from build123d import *

# Parameters (mm, degrees)
F0_W        = 2
F0_H        = 7
F1_DEPTH    = 8
F2_T1_DEPTH = 28


# Not quite as in the source:
# - a fillet or chamfer that OpenCascade refuses, or shapes differently, is made with other operations: its cross-section is extruded or revolved along the edge and cut away or added


with BuildPart() as f1:
    # F0 (on Front) → F1 (new body)
    with BuildSketch(Plane.XZ):
        with Locations((-3, 4)):
            Rectangle(F0_W, F0_H)
        Polygon((-2, 0.5), (-4, 0.5), (-4, -0.5), (4, -0.5), (4, 0.5), (2, 0.5), align=None)
        with Locations((3, 4)):
            Rectangle(F0_W, F0_H)
    extrude(amount=F1_DEPTH)

    # F2: fillet of radius 5 on 2 edges, made by hand

    # F2_s2 → F2_t1 (cut)
    with BuildSketch(Plane.XZ.offset(-10)):
        with BuildLine():
            ThreePointArc((-2, 3.5), (-2.527864045, 5.7360679775), (-4, 7.5))
            Line((-4, 7.5), (-2, 7.5))
            Line((-2, 7.5), (-2, 3.5))
        make_face()
        with BuildLine():
            ThreePointArc((4, 7.5), (2.527864045, 5.7360679775), (2, 3.5))
            Line((2, 3.5), (2, 7.5))
            Line((2, 7.5), (4, 7.5))
        make_face()
    extrude(amount=F2_T1_DEPTH, mode=Mode.SUBTRACT)


solid = f1.part
Here's how the part is built. I have some questions about the finished solid (model axes, mm). A direction names the side the tool comes from. Give positions to 0.01 mm unless a question says otherwise; leave off trailing zeros. Order: outer loops, then holes, each group sorted by start corner. A loop starts at its lowest first (then second) coordinate and runs counter-clockwise, first axis right, second up. Notation, with made-up numbers: (-11.75, 10.25) -> (7.25, 10.25) arc R17 cw to (7.25, 39.25) -> close; hole circle Ø2 at (-38.75, 42.5). An arc over 180 degrees is marked (long way). Use a Markdown table: item, result. Add a question column.
Item 1: If we mould it in two halves opening along X, with no side actions, what happens to faces 3 (the face through (4, -4, 3)), 4 (the face through (-4, -4, 4)), 5 (the face through (-2.513, -3.944, 5.707))? For each: pulls with the +X half, pulls with the -X half, needs draft (parallel to the pull), parting line crosses it, or undercut.
Item 2: Imagine slicing it at C-C on x = -1.75. Please give me the cut outline in (y, z), plus the area to 3 significant figures.
Item 3: Imagine slicing it at B-B on y = -0.75. Please give me the cut outline in (x, z), plus the area to 3 significant figures.
Item 4: Will these pins go through, and if not, where does the flat tip stop? pin 1 (3 mm diameter, centred on x = 2, y = -6.5, fed in from +Z); pin 2 (1.2 mm diameter, centred on x = -1, y = -5.5, fed in from +Z).
Item 5: I need wall thicknesses on line 1 (X direction, y = -1, z = 3.5); line 2 (Z direction, x = 0.5, y = -2.75); line 3 (X direction, y = -1.75, z = 6.25). Which ranges of each line are inside material? Lowest first, please.
Item 6: Imagine slicing it at A-A on z = 5.75. Please give me the cut outline in (x, y).
Item 7: For faces 1 (the face through (2.542, -3.944, 5.765)), 2 (the face through (-3, -8, 3)), which set-ups out of +Z, -Z, +X, -X, +Y, -Y let a thin tool reach every point of the face, with its end or its side?
Data:
| question | item | result |
|---|---|---|
| 1 | face 3 | pulls with the +X half |
| 1 | face 4 | pulls with the -X half |
| 1 | face 5 | undercut |
| 2 | outline | (-8, -0.5) -> (0, -0.5) -> (0, 0.5) -> (-8, 0.5) -> close |
| 2 | area | 8.00 mm² |
| 3 | outline | (-4, -0.5) -> (4, -0.5) -> (4, 7.5) arc R5 ccw to (2, 3.5) -> (2, 0.5) -> (-2, 0.5) -> (-2, 3.5) arc R5 ccw to (-4, 7.5) -> close |
| 3 | area | 31.2 mm² |
| 4 | pin 1 | stops at z = 7.07 |
| 4 | pin 2 | stops at z = 0.5 |
| 5 | line 1 | x = -4 to -2, 2 to 4 |
| 5 | line 2 | z = -0.5 to 0.5 |
| 5 | line 3 | x = -4 to -2.82, 2.82 to 4 |
| 6 | outline | (-4, -8) -> (-2.53, -8) -> (-2.53, 0) -> (-4, 0) -> close; (2.53, -8) -> (4, -8) -> (4, 0) -> (2.53, 0) -> close |
| 7 | face 1 | +Z, +Y, -Y |
| 7 | face 2 | +Z, -Z, +X, -X, -Y |
